Autodesk Inventor part; units mm, degrees
ref_plane "YZ Plane" through (0, 0, 0) normal (1, 0, 0) x (0, 1, 0)
ref_plane "XZ Plane" through (0, 0, 0) normal (0, 1, 0) x (-1, 0, 0)
ref_plane "XY Plane" through (0, 0, 0) normal (0, 0, 1) x (1, 0, 0)
sketch "Эскиз1" plane through (0, 0, 0) normal (0, 0, 1) x (1, 0, 0)
  circle A0 centre (0, 0) radius 5
  circle A1 centre (0, 0) radius 12.5
  arc A2 (-2.4853, 79.8323) -> (82.4853, 79.8323) centre (40, 65) ccw
  arc A3 (57.6777, 47.3223) -> (22.3223, 47.3223) centre (40, 65) ccw construction
  arc A4 (64.7487, 40.2513) -> (15.2513, 40.2513) centre (40, 65) ccw
  arc A5 (50.6066, 54.3934) -> (29.3934, 54.3934) centre (40, 65) ccw
  arc A6 (50.6066, 54.3934) -> (64.7487, 40.2513) centre (57.6777, 47.3223) ccw
  arc A7 (15.2513, 40.2513) -> (29.3934, 54.3934) centre (22.3223, 47.3223) ccw
  line L0 (40, 65) -> (57.6777, 47.3223) construction
  line L1 (40, 65) -> (65, 65) construction
  line L2 (40, 65) -> (22.3223, 47.3223) construction
  line L3 (-12.5, 0) -> (-5, 65)
  circle A8 centre (40, 140) radius 15
  arc A9 (65, 140) -> (15, 140) centre (40, 140) ccw
  line L4 (15, 140) -> (-3.8175, 75.2482)
  line L5 (65, 140) -> (83.8175, 75.2482)
  arc A10 (31.1612, 20.8766) -> (12.5, 0) centre (32.4788, 0.92) ccw
  dimension "d0" = 10
  dimension "d1" = 25
  dimension "d2" = 90
  dimension "d4" = 25
  dimension "d5" = 45
  dimension "d6" = 90
  dimension "d7" = 20
  dimension "d9" = 30
  dimension "d10" = 50
  dimension "d11" = 20
  dimension "d24" = 73.796
  dimension "d25" = 32.409
  dimension "d26" = 22.786
  dimension "d27" = 101.4868
  dimension "d28" = 65
  dimension "d29" = 74.2462
  dimension "d30" = 24.665
  dimension "d31" = 12.4176
  dimension "d32" = 75
  dimension "d33" = 24.0068
  dimension "d34" = 70.0415
  dimension "d35" = 64.0799
extrude "Выдавливание1" add sketch "Эскиз1" along normal blind 10 contours L3 A1 A10 | L3 A2 A10 A1
extrude "Выдавливание2" add sketch "Эскиз1" along normal blind 20 contours A2 L4 A9 L5
properties part number "LR3_2"
Could you check a few things on this model? Use its own coordinates, in mm. A direction names the side the tool comes from. Coordinates: 2 decimals unless noted, no trailing zeros. Loops run counter-clockwise (first coordinate to the right, second up) from the corner with the lowest first, then second, coordinate; pieces in that order, holes last.
1. Imagine slicing it at A-A (x = 40). Please give me the cut outline in (y, z), and give its area (3 significant figures).
2. Imagine slicing it at B-B (z = 15.75). Please give me the cut outline in (x, y), and give its area (3 significant figures).
3. We'd pull the mould along X, two halves only. Please class faces 4 (the face through (5.723, 108.077, 9.86)), 5 (the face through (29.55, 40.41, 9.86)), 6 (the face through (0.275, -12.497, 4.93)): released by +X, released by -X, zero draft, split by the parting line, or undercut.
4. I need wall thicknesses on L1, parallel to X at y = 66, z = 11.25; L2, parallel to Y at x = 40, z = 11.25; L3, parallel to X at y = 50.5, z = 17. Which ranges of each line are inside material? Lowest first, please.
5. For P1, Ø8, axis at x = 50.5, z = 12, coming from the -Y side; P2, Ø12, axis at y = 51, z = 14, coming from the +X side; P3, Ø4, axis at x = 39, z = 16, coming from the +Y side, each with a flat end and sliding along its axis, tell me the tip position at first contact or that it passes through.
6. For faces 1 (the face through (40, 80, 10)), 2 (the face through (-1, 18, 10)), 3 (the face through (58.57, 24.01, 9.86)), which set-ups out of +Z, -Z, +X, -X, +Y, -Y let a thin tool reach every point of the face, with its end or its side?
7. Imagine slicing it at D-D (z = 5.5). Please give me the cut outline in (x, y), and give its area (3 significant figures).
8. Imagine slicing it at C-C (x = 0). Please give me the cut outline in (y, z), and give its area (3 significant figures).
Computed values:
1. outline: (20, 0) - (80, 0) - (80, 20) - (20, 20) - close; (100, 0) - (125, 0) - (125, 20) - (100, 20) - close; (155, 0) - (165, 0) - (165, 20) - (155, 20) - close
1. area: 1,900 mm2
2. outline: (-3.82, 75.25) arc R45 ccw (long way) to (83.82, 75.25) - (65, 140) arc R25 ccw to (15, 140) - close; hole (15.25, 40.25) arc R10 ccw to (29.39, 54.39) arc R15 cw (long way) to (50.61, 54.39) arc R10 ccw to (64.75, 40.25) arc R35 ccw (long way) to start; hole circle Ø30 at (40, 140)
2. area: 6,160 mm2
3. face 4: released by -X
3. face 5: undercut
3. face 6: split by the parting line
4. L1: x = -4.99 to 5.01, 25.03 to 54.97, 74.99 to 84.99
4. L2: y = 20 to 80, 100 to 125, 155 to 165
4. L3: x = -2.6 to 8.14, 31.8 to 48.2, 71.86 to 82.6
5. P1: stops at y = 20.47
5. P2: stops at x = 84.28
5. P3: stops at y = 165
6. face 1: +Z, -Z
6. face 2: +Z, -X, -Y
6. face 3: +Z
7. outline: (-12.5, 0) arc R12.5 ccw to (12.5, 0) arc R20 cw to (31.16, 20.88) arc R45 ccw to (83.82, 75.25) - (65, 140) arc R25 ccw to (15, 140) - (-3.82, 75.25) arc R45 ccw to (-5, 65) - close; hole circle Ø10 at (0, 0); hole (15.25, 40.25) arc R10 ccw to (29.39, 54.39) arc R15 cw (long way) to (50.61, 54.39) arc R10 ccw to (64.75, 40.25) arc R35 ccw (long way) to start; hole circle Ø30 at (40, 140)
7. area: 7,420 mm2
8. outline: (-12.5, 0) - (-5, 0) - (-5, 10) - (-12.5, 10) - close; (5, 0) - (88.38, 0) - (88.38, 20) - (44.38, 20) - (44.38, 10) - (5, 10) - close
8. area: 1,350 mm2
